Check sheet for the modelled part. Datum: model origin and axes. Units: mm. A direction names the side the tool comes from. Round coordinates to 2 decimals unless told otherwise and drop trailing zeros. Loops run counter-clockwise (first coordinate to the right, second up) from the corner with the lowest first, then second, coordinate; pieces in that order, holes last. Notation, with made-up numbers: (-31, -26) -> (-6, -26) arc R18 ccw to (-6, -21) -> close; hole circle Ø5 at (68.25, -15.5). An arc over 180 degrees is marked (long way). Return JSON: item names as keys, results as strings.
from build123d import *

# Parameters (mm, degrees)
BOSS_EXTRUDE1_DEPTH       = 7.62
F_6_32_TAPPED_HOLE1_D     = 2.7051
F_6_32_TAPPED_HOLE1_DEPTH = 0.635
CUT_EXTRUDE1_REACH        = 9.62
SKETCH6_R                 = 2.159


with BuildPart() as part:
    # Sketch1 → Boss-Extrude1 (new body)
    with BuildSketch(Plane.XY):
        Polygon((-3.353873239, 6.85218662), (-3.353873239, -2.29181338), (4.266126761, -2.29181338), (4.266126761, 6.85218662), (3.631126761, 6.85218662), (3.631126761, -1.52981338), (-2.718873239, -1.52981338), (-2.718873239, 6.85218662), align=None)
    extrude(amount=BOSS_EXTRUDE1_DEPTH)

    # #6-32 Tapped Hole1
    with Locations(Plane.ZY.offset(3.353873239)):
        with Locations((3.81, 4.05818662)):
            Hole(F_6_32_TAPPED_HOLE1_D / 2, depth=F_6_32_TAPPED_HOLE1_DEPTH)

    # Sketch6 → Cut-Extrude1 (cut, up to next)
    with BuildSketch(Plane(origin=(4.266126761, 0, 0), x_dir=(0, 0, -1), z_dir=(1, 0, 0)), mode=Mode.PRIVATE) as cut_extrude1_sk1:
        with Locations((-3.81, 4.05818662)):
            Circle(SKETCH6_R)
    cut_extrude1_tool1 = extrude(cut_extrude1_sk1.sketch, amount=-CUT_EXTRUDE1_REACH, mode=Mode.PRIVATE) & part.part
    add(cut_extrude1_tool1.solids().sort_by_distance((4.266127, 4.058187, 3.81))[0], mode=Mode.SUBTRACT)


solid = part.part
Q1. Section check B-B (y = -0.5). Record the boundary of the cut face in (x, z), then the cut area to 3 significant figures.
Results list:
{"outline": "(-3.35, 0) -> (-2.72, 0) -> (-2.72, 7.62) -> (-3.35, 7.62) -> close; (3.63, 0) -> (4.27, 0) -> (4.27, 7.62) -> (3.63, 7.62) -> close", "area": "9.68 mm^2"}
Q2. Section check C-C (z = 2). Record the boundary of the cut face in (x, y).
Results list:
{"outline": "(-3.35, -2.29) -> (4.27, -2.29) -> (4.27, 2.88) -> (3.63, 2.88) -> (3.63, -1.53) -> (-2.72, -1.53) -> (-2.72, 6.85) -> (-3.35, 6.85) -> close; (3.63, 5.24) -> (4.27, 5.24) -> (4.27, 6.85) -> (3.63, 6.85) -> close"}
Q3. Section check D-D (y = 3.25). Record the boundary of the cut face in (x, z).
Results list:
{"outline": "(-3.35, 0) -> (-2.72, 0) -> (-2.72, 2.73) -> (-3.35, 2.73) -> close; (-3.35, 4.89) -> (-2.72, 4.89) -> (-2.72, 7.62) -> (-3.35, 7.62) -> close; (3.63, 0) -> (4.27, 0) -> (4.27, 1.81) -> (3.63, 1.81) -> close; (3.63, 5.81) -> (4.27, 5.81) -> (4.27, 7.62) -> (3.63, 7.62) -> close"}
Q4. Draft check along X on faces 1 (the flat face through (4.266, 1, 4)), 2 (the flat face through (0, -2, 0)), 3 (the flat face through (1, -1.53, 4)). Enter one of: released by +X, released by -X, zero draft, split by the parting line, or undercut.
Results list:
{"face 1": "released by +X", "face 2": "zero draft", "face 3": "undercut"}
Q5. Go/stop test with a flat-tipped pin: pin 1 (3 mm diameter, centred on x = 0.5, z = 6.5, fed in from +Y). Record where the tip stops, or that it passes through.
Results list:
{"pin 1": "y = -1.53"}
Q6. Section check A-A (z = 3.81). Record the boundary of the cut face in (x, y), then the cut area to 3 significant figures.
Results list:
{"outline": "(-3.35, -2.29) -> (4.27, -2.29) -> (4.27, 1.9) -> (3.63, 1.9) -> (3.63, -1.53) -> (-2.72, -1.53) -> (-2.72, 2.71) -> (-3.35, 2.71) -> close; (-3.35, 5.41) -> (-2.72, 5.41) -> (-2.72, 6.85) -> (-3.35, 6.85) -> close; (3.63, 6.22) -> (4.27, 6.22) -> (4.27, 6.85) -> (3.63, 6.85) -> close", "area": "12.0 mm^2"}
Q7. Tool access check on faces 4 (the cylindrical face through (3.953, 4.153, 5.967)), 5 (the cylindrical face through (-3.032, 5.199, 3.083)), 6 (the flat face through (3.631, 1.8, 2.9)). Record the directions out of +Z, -Z, +X, -X, +Y, -Y that give a thin tool (end or side, any length) a straight path to the whole face; none if there is none.
Results list:
{"face 4": "+X", "face 5": "+X, -X", "face 6": "+Z, -Z, +Y"}
Q8. Material ranges on line 1 (Y direction, x = 4.1, z = 3.81); line 2 (X direction, y = -0.25, z = 6.5); line 3 (Y direction, x = -0.5, z = 6), recorded low to high.
Results list:
{"line 1": "-2.29 to 1.9, 6.22 to 6.85", "line 2": "-3.35 to -2.72, 3.63 to 4.27", "line 3": "-2.29 to -1.53"}
